Can you work these out from the model? Positions are in its coordinate system, mm. Face numbers are marked on the shaded views. A direction names the side the tool comes from. Give positions to 0.01 mm unless a question says otherwise; leave off trailing zeros. Write each loop counter-clockwise with the first axis right and the second up, starting at its lowest first coordinate (ties: lowest second). Pieces come first, ordered by that corner, then holes.
```python
from build123d import *

# Parameters (mm, degrees)
SKETCH1_R      = 6
EXTRUDE1_DEPTH = 4.94
HOLE1_D        = 10.6635
HOLE1_DEPTH    = 0.823333333
SKETCH4_R      = 3.873625
EXTRUDE2_DEPTH = 0.823333333
HOLE2_D        = 10.6635
HOLE2_DEPTH    = 0.823333333
SKETCH7_R      = 3.873625
EXTRUDE3_DEPTH = 0.823333333
HOLE3_D        = 5.9975
HOLE3_DEPTH    = 4.94
CHAMFER1_SIZE  = 0.247


with BuildPart() as part:
    # Sketch1 → Extrude1 (new body)
    with BuildSketch(Plane.XY.offset(4.94)):
        Circle(SKETCH1_R)
    extrude(amount=-EXTRUDE1_DEPTH)

    # Hole1
    with Locations(Plane.XY.offset(4.94)):
        with Locations((0, 0)):
            Hole(HOLE1_D / 2, depth=HOLE1_DEPTH)

    # Sketch4 → Extrude2 (add)
    with BuildSketch(Plane.XY.offset(4.116666667)):
        Circle(SKETCH4_R)
    extrude(amount=EXTRUDE2_DEPTH)

    # Hole2
    with Locations(Plane(origin=(0, 0, 0), x_dir=(-1, 0, 0), z_dir=(0, 0, -1))):
        with Locations((0, 0)):
            Hole(HOLE2_D / 2, depth=HOLE2_DEPTH)

    # Sketch7 → Extrude3 (add)
    with BuildSketch(Plane(origin=(0, 0, 0.823333333), x_dir=(-1, 0, 0), z_dir=(0, 0, -1))):
        Circle(SKETCH7_R)
    extrude(amount=EXTRUDE3_DEPTH)

    # Hole3
    with Locations(Plane(origin=(0, 0, 0), x_dir=(-1, 0, 0), z_dir=(0, 0, -1))):
        with Locations((0, 0)):
            Hole(HOLE3_D / 2, depth=HOLE3_DEPTH)

    # Chamfer1
    chamfer1_edges = [part.edges().sort_by_distance(p)[0] for p in [
        (-6, 0, 4.94),
        (-2.99875, 0, 0),
        (-2.99875, 0, 4.94),
        (-6, 0, 0),
    ]]
    chamfer(chamfer1_edges, length=CHAMFER1_SIZE)


solid = part.part
```
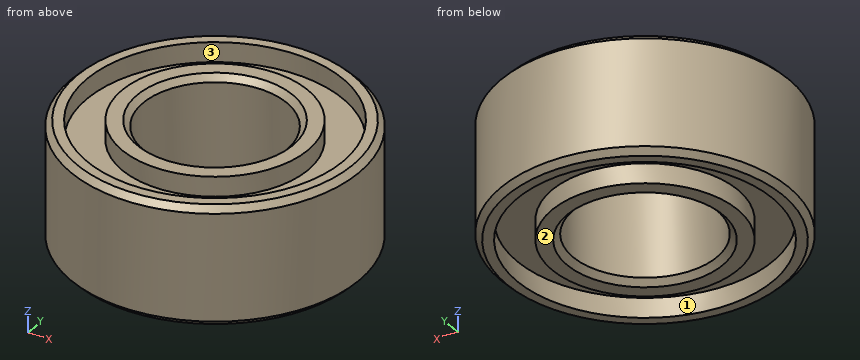
1) For the marked faces 1, 2 and 3, which set-ups out of +Z, -Z, +X, -X, +Y, -Y let a thin tool reach every point of the face, with its end or its side?
Values follow:
face 1: -Z
face 2: -Z, +X, -X, +Y, -Y
face 3: +Z
2) Please list where these lines run through material, in increasing order: L1, parallel to Y at x = 0, z = 4.4; L2, parallel to Y at x = -3.25, z = 4.3; L3, parallel to X at y = 1.75, z = 0.5.
Values follow:
L1: y = -6 to -5.33, -3.87 to -3, 3 to 3.87, 5.33 to 6
L2: y = -5.04 to -4.23, -2.11 to 2.11, 4.23 to 5.04
L3: x = -5.74 to -5.04, -3.46 to -2.44, 2.44 to 3.46, 5.04 to 5.74
3) Suppose I cut it at C-C on z = 3.6. Write out the boundary of the cut face in (x, y).
Values follow:
outline: circle Ø12 at (0, 0); hole circle Ø6 at (0, 0)
4) For pin 1 Ø4 at (x, y) = (-1.5, -1) entering from +Z; pin 2 Ø3.5 at (x, y) = (0, 0) entering from -Z; pin 3 Ø1.5 at (x, z) = (2, 1) entering from +Y, each with a flat end and sliding along its axis, tell me the tip position at first contact or that it passes through.
Values follow:
pin 1: stops at z = 4.94
pin 2: passes through
pin 3: stops at y = 5.87
